For this review, take the finished solid that the model builds, in its own axes (mm). Coordinates: 2 decimals unless noted, no trailing zeros. Loops run counter-clockwise (first coordinate to the right, second up) from the corner with the lowest first, then second, coordinate; pieces in that order, holes last. Notation, with made-up numbers: M 48.25,6.25 L 81.25,6.25 A19 ccw 81.25,38.25 Z; hole C 5.25,50 d1. An arc over 180 degrees is marked long. Answer as a JSON object with one key per item and string values. Group by question number.
Item 1: Add section B-B (y = -8). State the section outline as (x, z) points, then the cut area to 3 significant figures.
Item 2: Add section A-A (x = -49). State the section outline as (y, z) points, then the cut area to 3 significant figures.
Item 3: Add section C-C (z = 30). State the section outline as (x, y) points.
Item 4: Wall thickness on L1, parallel to Z at x = -40, y = -5.5; L2, parallel to Z at x = -46, y = -7.25; L3, parallel to X at y = -3.75, z = 17.5: over which ranges is each line inside the solid? List them lowest first. Write a range as from..to.
from build123d import *

# Parameters (mm, degrees)
F0_W     = 40
F0_H     = 30
F1_DEPTH = 10
F2_R     = 15
F3_DEPTH = 10.001


with BuildPart() as f1:
    # F0 (on Front) → F1 (new body)
    with BuildSketch(Plane.XZ):
        with Locations((-20, 15)):
            Rectangle(F0_W, F0_H)
        with Locations((-60, 15)):
            Rectangle(F0_W, F0_H)
        with Locations((-20, 45)):
            Rectangle(F0_W, F0_H)
        with Locations((-60, 45)):
            Rectangle(F0_W, F0_H)
    extrude(amount=F1_DEPTH)

    # F2 (on face) → F3 (cut, through all)
    with BuildSketch(Plane.XZ.offset(10)):
        with Locations((-40, 30)):
            Circle(F2_R)
    extrude(amount=-F3_DEPTH, mode=Mode.SUBTRACT)


solid = f1.part
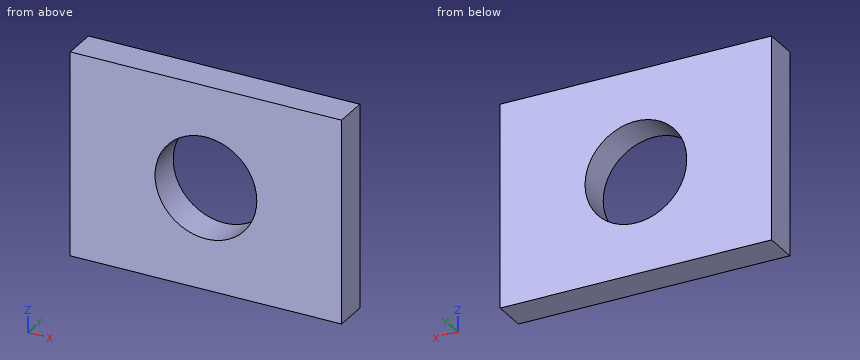
From the geometry:
{
 "1": {"outline": "M -80,0 L 0,0 L 0,60 L -80,60 Z; hole C -40,30 d30", "area": "4,090 mm²"},
 "2": {"outline": "M -10,0 L 0,0 L 0,18 L -10,18 Z; M -10,42 L 0,42 L 0,60 L -10,60 Z", "area": "360 mm²"},
 "3": {"outline": "M -80,-10 L -55,-10 L -55,0 L -80,0 Z; M -25,-10 L 0,-10 L 0,0 L -25,0 Z"},
 "4": {"L1": "z = 0..15, 45..60", "L2": "z = 0..16.25, 43.75..60", "L3": "x = -80..-48.29, -31.71..0"}
}
